Read the model definition and answer for the solid it produces. Units are mm, in the model's axes. A direction names the side the tool comes from. Coordinates: 2 decimals unless noted, no trailing zeros. Loops run counter-clockwise (first coordinate to the right, second up) from the corner with the lowest first, then second, coordinate; pieces in that order, holes last.
from build123d import *

# Parameters (mm, degrees)
SKETCH1_W           = 34
SKETCH1_H           = 30
SKETCH1_R           = 2.25
BOSS_EXTRUDE1_DEPTH = 5
SKETCH2_W           = 34
SKETCH2_H           = 5
BOSS_EXTRUDE2_DEPTH = 10
SKETCH3_W           = 34
SKETCH3_H           = 5
BOSS_EXTRUDE3_DEPTH = 20
SKETCH4_R           = 2.5
CUT_EXTRUDE1_DEPTH  = 20


with BuildPart() as part:
    # Sketch1 → Boss-Extrude1 (new body)
    with BuildSketch(Plane.XY):
        with Locations((17, 15)):
            Rectangle(SKETCH1_W, SKETCH1_H)
        with Locations((4.75, 25.25)):
            Circle(SKETCH1_R, mode=Mode.SUBTRACT)
        with Locations((29.25, 25.25)):
            Circle(SKETCH1_R, mode=Mode.SUBTRACT)
        with Locations((29.25, 4.75)):
            Circle(SKETCH1_R, mode=Mode.SUBTRACT)
        with Locations((4.75, 4.75)):
            Circle(SKETCH1_R, mode=Mode.SUBTRACT)
    extrude(amount=BOSS_EXTRUDE1_DEPTH)

    # Sketch2 → Boss-Extrude2 (add)
    with BuildSketch(Plane(origin=(0, 30, 0), x_dir=(1, 0, 0), z_dir=(0, 1, 0))):
        with Locations((17, -2.5)):
            Rectangle(SKETCH2_W, SKETCH2_H)
    extrude(amount=BOSS_EXTRUDE2_DEPTH)

    # Sketch3 → Boss-Extrude3 (add)
    with BuildSketch(Plane.XY.offset(5)):
        with Locations((17, 37.5)):
            Rectangle(SKETCH3_W, SKETCH3_H)
    extrude(amount=BOSS_EXTRUDE3_DEPTH)

    # Sketch4 → Cut-Extrude1 (cut)
    with BuildSketch(Plane(origin=(0, 40, 0), x_dir=(1, 0, 0), z_dir=(0, 1, 0))):
        with Locations(Location((8, -13, 0), (0, 0, 270))):
            Circle(SKETCH4_R)
        with Locations(Location((26, -13, 0), (0, 0, 270))):
            Circle(SKETCH4_R)
    extrude(amount=-CUT_EXTRUDE1_DEPTH, mode=Mode.SUBTRACT)


solid = part.part
Q1. A cutting plane is placed at B-B (x = 4.75). Give the vertices of the cut face in (y, z).
Findings below:
outline: (0, 0) - (2.5, 0) - (2.5, 5) - (0, 5) - close; (7, 0) - (23, 0) - (23, 5) - (7, 5) - close; (27.5, 0) - (40, 0) - (40, 25) - (35, 25) - (35, 5) - (27.5, 5) - close
Q2. Flat-ended cylindrical pins translate along their axes: pin 1 Ø6 at (x, z) = (17, 10.5) entering from -Y; pin 2 Ø5 at (x, y) = (29.25, 25.25) entering from +Z. Find the tip coordinate at first contact, or state that the pin passes through.
Findings below:
pin 1: stops at y = 35
pin 2: stops at z = 5
Q3. Straight lines are drawn through the part: probe 1 along Y at (x, z) = (29.25, 1.8); probe 2 along X at (y, z) = (36.55, 13); probe 3 along Z at (x, y) = (15.5, 30.5). For each, find the intervals that lie inside material, in ascending order.
Findings below:
probe 1: y = 0 to 2.5, 7 to 23, 27.5 to 40
probe 2: x = 0 to 5.5, 10.5 to 23.5, 28.5 to 34
probe 3: z = 0 to 5
Q4. Which of the six approach directions +Z, -Z, +X, -X, +Y, -Y give full straight-line access (tool end or side, diameter ignored) to faces 1 (the face through (17, 35, 15)), 2 (the face through (17, 38, 25))?
Findings below:
face 1: +Z, +X, -X, -Y
face 2: +Z, +X, -X, +Y, -Y
Q5. A cutting plane is placed at D-D (y = 37). Give the vertices of the cut face in (x, z), then the cut area to 3 significant figures.
Findings below:
outline: (0, 0) - (34, 0) - (34, 25) - (0, 25) - close; hole circle Ø5 at (8, 13); hole circle Ø5 at (26, 13)
area: 811 mm2
Q6. A cutting plane is placed at C-C (x = 25). Give the vertices of the cut face in (y, z), then the cut area to 3 significant figures.
Findings below:
outline: (0, 0) - (40, 0) - (40, 10.71) - (35, 10.71) - (35, 5) - (0, 5) - close; (35, 15.29) - (40, 15.29) - (40, 25) - (35, 25) - close
area: 277 mm2
Q7. Determine the mould class of faces 3 (the face through (17, 17, 5)), 4 (the face through (0, 26, 4)), 5 (the face through (6.5, 37.5, 11)) for opening direction X: +X half, -X half, draft (parallel to the pull), parting line (faces both ways), or undercut.
Findings below:
face 3: draft
face 4: -X half
face 5: undercut
Q8. A cutting plane is placed at A-A (y = 25.25). Give the vertices of the cut face in (x, z).
Findings below:
outline: (0, 0) - (2.5, 0) - (2.5, 5) - (0, 5) - close; (7, 0) - (27, 0) - (27, 5) - (7, 5) - close; (31.5, 0) - (34, 0) - (34, 5) - (31.5, 5) - close
